from build123d import *

# Parameters (mm, degrees)
SKETCH_1_R      = 4.1
EXTRUDE_1_DEPTH = 12
CHAMFER_1_SIZE  = 20
FILLET_1_R      = 10
CHAMFER_2_SIZE  = 2


with BuildPart() as part:
    # 草图1 → 凸台-拉伸1 (new body)
    with BuildSketch(Plane.XY):
        Polygon((-140, -10), (-140, -30), (-120, -30), (-120, -10), (10, -10), (65, -10), (65, -30), (85, -30), (85, 10), (10, 10), (-120, 10), (-140, 10), align=None)
        Circle(SKETCH_1_R, mode=Mode.SUBTRACT)
        with Locations((-50, 0)):
            Circle(SKETCH_1_R, mode=Mode.SUBTRACT)
        with Locations((-130, 0)):
            Circle(SKETCH_1_R, mode=Mode.SUBTRACT)
        with Locations((-130, -20)):
            Circle(SKETCH_1_R, mode=Mode.SUBTRACT)
        with Locations((75, 0)):
            Circle(SKETCH_1_R, mode=Mode.SUBTRACT)
        with Locations((75, -20)):
            Circle(SKETCH_1_R, mode=Mode.SUBTRACT)
    extrude(amount=EXTRUDE_1_DEPTH)

    # 倒角1
    chamfer_1_edges = [part.edges().sort_by_distance(p)[0] for p in [
        (65, -10, 6),
        (-120, -10, 6),
    ]]
    chamfer(chamfer_1_edges, length=CHAMFER_1_SIZE - 0.0001)  # a hair under: the kernel refuses the full size

    # 圆角1
    fillet_1_edges = [part.edges().sort_by_distance(p)[0] for p in [
        (-100.0001, -10, 6),
        (45.0001, -10, 6),
    ]]
    fillet(fillet_1_edges, radius=FILLET_1_R)

    # 倒角2
    chamfer_2_edges = [part.edges().sort_by_distance(p)[0] for p in [
        (-140, -30, 6),
        (-140, 10, 6),
        (85, 10, 6),
        (85, -30, 6),
    ]]
    chamfer(chamfer_2_edges, length=CHAMFER_2_SIZE)


solid = part.part
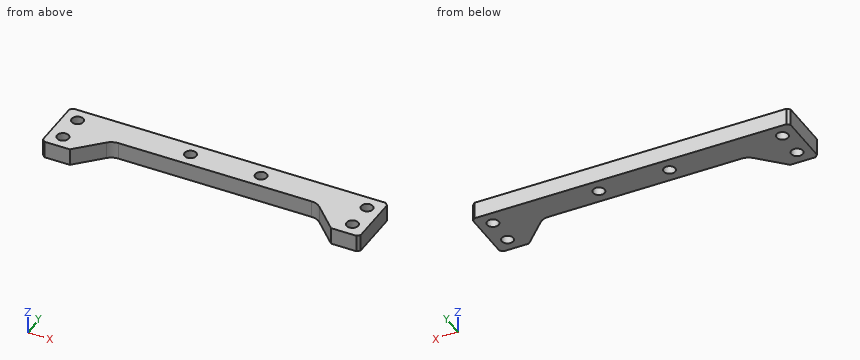
For this review, take the finished solid that the model builds, in its own axes (mm). Give positions to 0.01 mm unless a question says otherwise; leave off trailing zeros. Loops run counter-clockwise (first coordinate to the right, second up) from the corner with the lowest first, then second, coordinate; pieces in that order, holes last. Notation, with made-up numbers: M -5,-32.5 L 23,-32.5 A18 cw 23,-4.5 Z; hole C 40,-29 d5. An arc over 180 degrees is marked long. Answer as a JSON object with one key per item and string values. Group by question number.
Q1. Insertion check: P1, Ø2, axis at x = -111.5, z = 9.5, coming from the -Y side; P2, Ø6, axis at x = -19.5, z = 6.5, coming from the -Y side. Each pin has a flat end and moves straight along its axis. Give the tip position at first contact, or say it passes through.
Q2. Add section B-B on y = 0. Give the boundary of the cut face in (x, z).
Q3. Add section A-A on x = 75. Give the boundary of the cut face in (y, z).
Q4. Add section C-C on z = 9. Give the number of separate pieces and of enclosed holes in the cut face, and give its area (3 significant figures).
Q5. Add section D-D on x = 0. Give the boundary of the cut face in (y, z).
Q6. For probe 1 along Y at (x, z) = (-130, 7.75); probe 2 along Y at (x, z) = (-50, 3.75); probe 3 along Y at (x, z) = (-58, 1.25), list the stretches that pass through material, from the lowest coordinate up. Write a range as [from, to].
Checked values:
{
 "1": {"P1": "y = -22.5", "P2": "y = -10"},
 "2": {"outline": "M -140,0 L -134.1,0 L -134.1,12 L -140,12 Z; M -125.9,0 L -54.1,0 L -54.1,12 L -125.9,12 Z; M -45.9,0 L -4.1,0 L -4.1,12 L -45.9,12 Z; M 4.1,0 L 70.9,0 L 70.9,12 L 4.1,12 Z; M 79.1,0 L 85,0 L 85,12 L 79.1,12 Z"},
 "3": {"outline": "M -30,0 L -24.1,0 L -24.1,12 L -30,12 Z; M -15.9,0 L -4.1,0 L -4.1,12 L -15.9,12 Z; M 4.1,0 L 10,0 L 10,12 L 4.1,12 Z"},
 "4": {"separate pieces": "1", "enclosed holes": "6", "area": "5,380 mm²"},
 "5": {"outline": "M -10,0 L -4.1,0 L -4.1,12 L -10,12 Z; M 4.1,0 L 10,0 L 10,12 L 4.1,12 Z"},
 "6": {"probe 1": "[-30, -24.1], [-15.9, -4.1], [4.1, 10]", "probe 2": "[-10, -4.1], [4.1, 10]", "probe 3": "[-10, 10]"}
}
